Autodesk Inventor part; units mm, degrees
ref_plane "YZ Plane" through (0, 0, 0) normal (1, 0, 0) x (0, 1, 0)
ref_plane "XZ Plane" through (0, 0, 0) normal (0, 1, 0) x (-1, 0, 0)
ref_plane "XY Plane" through (0, 0, 0) normal (0, 0, 1) x (1, 0, 0)
sketch "Sketch1" plane through (0, 0, 0) normal (0, 1, 0) x (-1, 0, 0)
  line L0 (-13.5, -14) -> (-32.4622, -7.0983)
  line L1 (-13.5, -14) -> (-10.5, -14)
  line L2 (-10.5, -14) -> (-10.5, 1)
  line L3 (-10.5, 1) -> (-13.5, 1)
  line L4 (-13.5, 1) -> (-13.5, 16)
  line L5 (-13.5, 16) -> (-10.5, 16)
  line L6 (-10.5, 16) -> (-10.5, 31)
  line L7 (-10.5, 31) -> (-13.5, 31)
  line L8 (-13.5, 45) -> (-13.5, 31)
  line L9 (-13.5, 16) -> (-13.5, 1)
  line L10 (-32.4622, -7.0983) -> (-35.2813, -6.0723)
  line L11 (-35.2813, -6.0723) -> (-30.151, 8.0231)
  line L12 (-30.151, 8.0231) -> (-27.3319, 6.9971)
  line L13 (-27.3319, 6.9971) -> (-22.2016, 21.0925)
  line L14 (-22.2016, 21.0925) -> (-25.0207, 22.1185)
  line L15 (-25.0207, 22.1185) -> (-19.8904, 36.2139)
  line L16 (-19.8904, 36.2139) -> (-17.0713, 35.1879)
  line L17 (-13.5, 45) -> (-17.0713, 35.1879)
  line L18 (-22.2016, 21.0925) -> (-27.3319, 6.9971)
  point P0 (0, 0)
  dimension "d0" = 3
  dimension "d1" = 15
  dimension "d2" = 15
  dimension "d3" = 15
  dimension "d4" = 15
  dimension "d5" = 15
  dimension "d6" = 15
  dimension "d7" = 2.8191
extrude "Extrusion1" add sketch "Sketch1" along normal blind 3
properties part number "do_sensor_2"
Can you work these out from the model? Positions are in its coordinate system, mm. A direction names the side the tool comes from. Coordinates: 2 decimals unless noted, no trailing zeros. Order: outer loops, then holes, each group sorted by start corner. A loop starts at its lowest first (then second) coordinate and runs counter-clockwise, first axis right, second up.
1. If we section it at A-A (y = 1.6): Please give me the cut outline in (x, z), then the cut area to 3 significant figures.
2. For faces 1 (the face through (10.5, 1, 23)), 2 (the face through (12, 1, 1)), 3 (the face through (18.501, 1.479, 35.708)), 4 (the face through (12, 1, 31)), 5 (the face through (20, 0, 9)), which set-ups out of +Z, -Z, +X, -X, +Y, -Y let a thin tool reach every point of the face, with its end or its side?
3. I need wall thicknesses on line 1 (Z direction, x = 11.5, y = 0.5); line 2 (X direction, y = 0.75, z = -5.5); line 3 (Z direction, x = 28, y = 0.3). Which ranges of each line are inside material? Lowest first, please.
4. I'm going to push flat-ended pins straight in: pin 1 (1 mm diameter, centred on x = 27.5, y = 1, fed in from -Z); pin 2 (1.5 mm diameter, centred on y = 1.5, z = 7.5, fed in from -X); pin 3 (0.9 mm diameter, centred on x = 11.5, y = 1, fed in from +Z). Where does each tip first touch, or does it pass through?
5. If we section it at C-C (x = 31): Please give me the cut outline in (y, z).
6. If we section it at B-B (z = -2.5): Please give me the cut outline in (x, y), then the cut area to 3 significant figures.
7. Thinking about a two-plate mould opening in Z: for faces 6 (the face through (28.761, 1.479, 7.517)), 7 (the face through (23.6, 1.5, 21.6)), 8 (the face through (13.5, 1, 38)), which applies, +Z half, -Z half, draft (parallel to the pull), parting line (faces both ways), or undercut?
Entries:
1. outline: (10.5, -14) - (13.5, -14) - (32.46, -7.1) - (35.28, -6.07) - (30.15, 8.02) - (27.33, 7) - (22.2, 21.09) - (25.02, 22.12) - (19.89, 36.21) - (17.07, 35.19) - (13.5, 45) - (13.5, 31) - (10.5, 31) - (10.5, 16) - (13.5, 16) - (13.5, 1) - (10.5, 1) - close
1. area: 739 mm2
2. face 1: +Z, -Z, -X, +Y, -Y
2. face 2: -X, +Y, -Y
2. face 3: +Z, +Y, -Y
2. face 4: +Z, -X, +Y, -Y
2. face 5: +Z, -Z, +X, -X, -Y
3. line 1: z = -14 to 1, 16 to 31
3. line 2: x = 10.5 to 35.07
3. line 3: z = -8.72 to 7.24
4. pin 1: stops at z = -9.09
4. pin 2: stops at x = 13.5
4. pin 3: stops at z = 31
5. outline: (0, -7.63) - (3, -7.63) - (3, 5.69) - (0, 5.69) - close
6. outline: (10.5, 0) - (33.98, 0) - (33.98, 3) - (10.5, 3) - close
6. area: 70.4 mm2
7. face 6: +Z half
7. face 7: undercut
7. face 8: draft
